from build123d import *

# Parameters (mm, degrees)
F1_DEPTH       = 25
F2_DEPTH       = 25
F3_DEPTH       = 25
F5_START       = -25
F5_DEPTH       = 25.001
F6_DEPTH       = 25
F7_DEPTH       = 50.001
F8_R           = 7.5
F9_DEPTH       = 25
F10_R          = 2.5
F11_DEPTH      = 25
F11_DEPTH_BACK = 25


with BuildPart() as f1:
    # F0 (on Front) → F1 (new body)
    with BuildSketch(Plane.XZ):
        with BuildLine():
            ThreePointArc((-38.6520479365, -14.6969384567), (-26.165214956, -11.6189500386), (-20.6520479365, 0))
            ThreePointArc((-20.6520479365, 0), (-26.165214956, 11.6189500386), (-38.6520479365, 14.6969384567))
            ThreePointArc((-38.6520479365, 14.6969384567), (-50.6520479365, 0), (-38.6520479365, -14.6969384567))
        make_face()
        with BuildLine():
            ThreePointArc((-38.6520479365, 14.6969384567), (-26.165214956, 11.6189500386), (-20.6520479365, 0))
            ThreePointArc((-20.6520479365, 0), (-26.165214956, -11.6189500386), (-38.6520479365, -14.6969384567))
            Line((-38.6520479365, -14.6969384567), (33.3479520635, -29.3938769134))
            ThreePointArc((33.3479520635, -29.3938769134), (9.3479520635, 0), (33.3479520635, 29.3938769134))
            Line((33.3479520635, 29.3938769134), (-38.6520479365, 14.6969384567))
        make_face()
        with BuildLine():
            ThreePointArc((69.3479520635, 0), (58.3216180245, 23.2379000772), (33.3479520635, 29.3938769134))
            ThreePointArc((33.3479520635, 29.3938769134), (9.3479520635, 0), (33.3479520635, -29.3938769134))
            ThreePointArc((33.3479520635, -29.3938769134), (58.3216180245, -23.2379000772), (69.3479520635, 0))
        make_face()
    extrude(amount=F1_DEPTH)

    # F0 (on Front) → F2 (join)
    with BuildSketch(Plane.XZ):
        with BuildLine():
            ThreePointArc((69.3479520635, 0), (58.3216180245, 23.2379000772), (33.3479520635, 29.3938769134))
            ThreePointArc((33.3479520635, 29.3938769134), (9.3479520635, 0), (33.3479520635, -29.3938769134))
            ThreePointArc((33.3479520635, -29.3938769134), (58.3216180245, -23.2379000772), (69.3479520635, 0))
        make_face()
    extrude(amount=F2_DEPTH)

    # F0 (on Front) → F3 (join)
    with BuildSketch(Plane.XZ):
        with BuildLine():
            ThreePointArc((69.3479520635, 0), (58.3216180245, 23.2379000772), (33.3479520635, 29.3938769134))
            ThreePointArc((33.3479520635, 29.3938769134), (9.3479520635, 0), (33.3479520635, -29.3938769134))
            ThreePointArc((33.3479520635, -29.3938769134), (58.3216180245, -23.2379000772), (69.3479520635, 0))
        make_face()
    extrude(amount=-F3_DEPTH)

    # F1_face (on face) → F5 (cut)
    with BuildSketch(Plane(origin=(15.2359623928, -25, 0), x_dir=(1, 0, 0), z_dir=(0, -1, 0)).offset(F5_START)):
        with BuildLine():
            Line((18.1119896706, 29.3938769134), (-53.8880103294, 14.6969384567))
            ThreePointArc((-53.8880103294, 14.6969384567), (-65.8880103294, 0), (-53.8880103294, -14.6969384567))
            Line((-53.8880103294, -14.6969384567), (18.1119896706, -29.3938769134))
            ThreePointArc((18.1119896706, -29.3938769134), (54.1119896706, 0), (18.1119896706, 29.3938769134))
        make_face()
    extrude(amount=-F5_DEPTH, mode=Mode.SUBTRACT)

    # F0 (on Front) → F6 (join)
    with BuildSketch(Plane.XZ):
        with BuildLine():
            ThreePointArc((69.3479520635, 0), (58.3216180245, 23.2379000772), (33.3479520635, 29.3938769134))
            ThreePointArc((33.3479520635, 29.3938769134), (9.3479520635, 0), (33.3479520635, -29.3938769134))
            ThreePointArc((33.3479520635, -29.3938769134), (58.3216180245, -23.2379000772), (69.3479520635, 0))
        make_face()
    extrude(amount=-F6_DEPTH)

    # F4 (on face) → F7 (cut, through all)
    with BuildSketch(Plane(origin=(0, 25, 0), x_dir=(-1, 0, 0), z_dir=(0, 1, 0))):
        Polygon((-18.48410815, -12.1983237636), (-18.48410815, 11.8132381481), (-39.2787307501, 23.8190191039), (-60.0733533502, 11.8132381481), (-60.0733533502, -12.1983237636), (-39.2787307501, -24.2041047195), align=None)
    extrude(amount=-F7_DEPTH, mode=Mode.SUBTRACT)

    # F8 (on face) → F9 (cut)
    with BuildSketch(Plane.XZ):
        with Locations((-36.0623635352, 0)):
            Circle(F8_R)
    extrude(amount=F9_DEPTH, mode=Mode.SUBTRACT)

    # F10 (on Top) → F11 (cut, two sides)
    with BuildSketch(Plane.XY) as f11_sk:
        with Locations((-38.1520479365, -12.5)):
            Circle(F10_R)
    extrude(amount=-F11_DEPTH, mode=Mode.SUBTRACT)
    extrude(f11_sk.sketch, amount=F11_DEPTH_BACK, mode=Mode.SUBTRACT)


solid = f1.part
Here's how the part is built. I have some questions about the finished solid (model axes, mm). A direction names the side the tool comes from. Round coordinates to 2 decimals unless told otherwise and drop trailing zeros. Order: outer loops, then holes, each group sorted by start corner. A loop starts at its lowest first (then second) coordinate and runs counter-clockwise, first axis right, second up. Notation, with made-up numbers: (-5.5, -20) -> (24.5, -20) arc R11 ccw to (24.5, -2) -> close; hole circle Ø5 at (57.5, -31). An arc over 180 degrees is marked (long way). Return JSON: item names as keys, results as strings.
Q1. If we section it at B-B on y = -21.5: List the corners of the cut face in (x, z) for me, plus the area to 3 significant figures.
Filled sheet:
{"outline": "(-38.65, -14.7) -> (33.35, -29.39) arc R30 ccw (long way) to (33.35, 29.39) -> (-38.65, 14.7) arc R15 ccw to start; hole circle Ø15 at (-36.06, 0); hole (18.48, -12.2) -> (39.28, -24.2) -> (60.07, -12.2) -> (60.07, 11.81) -> (39.28, 23.82) -> (18.48, 11.81) -> close", "area": "3,540 mm^2"}
Q2. Which directions (+Z, -Z, +X, -X, +Y, -Y) give clear straight access to the entire face, cutting with the end or side of a thin tool? Please do faces 1 (the flat face through (-3.16, -12.32, -21.94)), 2 (the flat face through (29.027, 0.35, -18.285)).
Filled sheet:
{"face 1": "-Z, -X, +Y, -Y", "face 2": "+Y, -Y"}
Q3. If we section it at A-A on y = 10.5: List the corners of the cut face in (x, z) for me, plus the area to 3 significant figures.
Filled sheet:
{"outline": "circle Ø60 at (39.35, 0); hole (18.48, -12.2) -> (39.28, -24.2) -> (60.07, -12.2) -> (60.07, 11.81) -> (39.28, 23.82) -> (18.48, 11.81) -> close", "area": "1,330 mm^2"}
Q4. If we section it at D-D on z = -21: List the corners of the cut face in (x, y) for me, plus the area to 3 significant figures.
Filled sheet:
{"outline": "(-7.77, -25) -> (33.73, -25) -> (33.73, 25) -> (17.92, 25) -> (17.92, 0) -> (-7.77, 0) -> close; (44.83, -25) -> (60.77, -25) -> (60.77, 25) -> (44.83, 25) -> close", "area": "2,230 mm^2"}
Q5. If we mould it in two halves opening along Y, with no side actions, what happens to faces 3 (the flat face through (28.736, 0.35, 17.732)), 4 (the cylindrical face through (-40.65, -12.39, 10.55)), 5 (the flat face through (9, -25, 0))? For each: released by +Y, released by -Y, zero draft, split by the parting line, or undercut.
Filled sheet:
{"face 3": "zero draft", "face 4": "undercut", "face 5": "released by -Y"}
Q6. If we section it at C-C on x = 50: List the corners of the cut face in (y, z) for me.
Filled sheet:
{"outline": "(-25, -28.05) -> (25, -28.05) -> (25, -18.01) -> (-25, -18.01) -> close; (-25, 17.63) -> (25, 17.63) -> (25, 28.05) -> (-25, 28.05) -> close"}
Q7. I need wall thicknesses on line 1 along X through (y, z) = (-12.5, -11.5); line 2 along Y through (x, z) = (-20, -11.5); line 3 along X through (y, z) = (-12.5, -11.75). Which ranges of each line are inside material? Lowest first, please. Write a range as from..to.
Filled sheet:
{"line 1": "x = -45.28..-40.65, -35.65..18.48, 60.07..67.06", "line 2": "y = -25..0", "line 3": "x = -44.98..-40.65, -35.65..18.48, 60.07..66.95"}
Q8. For pin 1 Ø6 at (x, y) = (-38.15, -12.5) entering from +Z; pin 2 Ø6 at (x, y) = (21, 11) entering from -Z; pin 3 Ø8 at (x, y) = (-38.15, -12.5) entering from -Z, each with a flat end and sliding along its axis, tell me the tip position at first contact or that it passes through.
Filled sheet:
{"pin 1": "stops at z = 15.41", "pin 2": "stops at z = -25.78", "pin 3": "stops at z = -15.62"}
